The model under review builds one solid part; all positions refer to its coordinate system, in mm. A direction names the side the tool comes from. Give positions to 0.01 mm unless a question says otherwise; leave off trailing zeros. Write each loop counter-clockwise with the first axis right and the second up, starting at its lowest first coordinate (ties: lowest second). Pieces come first, ordered by that corner, then holes. Notation, with made-up numbers: (77.25, 44.25) - (113.25, 44.25) arc R19 cw to (113.25, 58.25) - close; hole circle Ø2 at (-8, 55). An arc over 180 degrees is marked (long way). Write item = value, one per line.
```python
from build123d import *

# Parameters (mm, degrees)
SALIENTE_EXTRUIR1_DEPTH                              = 10
PERFORADOR_PARA_ROSCAR_PARA_MACHO_DE_2_COUNT         = 2
PERFORADOR_PARA_ROSCAR_PARA_MACHO_DE_2_PITCH         = 50
PERFORADOR_PARA_ROSCAR_PARA_MACHO_DE_3_COUNT         = 2
PERFORADOR_PARA_ROSCAR_PARA_MACHO_DE_3_PITCH         = 114.274917137
PERFORADOR_PARA_ROSCAR_PARA_MACHO_DE_4_COUNT         = 2
PERFORADOR_PARA_ROSCAR_PARA_MACHO_DE_4_PITCH         = 25
PERFORADOR_PARA_ROSCAR_PARA_MACHO_DE_5_A_COUNT       = 2
PERFORADOR_PARA_ROSCAR_PARA_MACHO_DE_5_A_PITCH       = 50
PERFORADOR_PARA_ROSCAR_PARA_MACHO_DE_6_COUNT         = 2
PERFORADOR_PARA_ROSCAR_PARA_MACHO_DE_6_PITCH         = 24.875395913
REFRENTADO_PARA_TORNILLO_TAP_N_CON_CABEZ_D           = 5.3
REFRENTADO_PARA_TORNILLO_TAP_N_CON_CABEZ_CSINK_D     = 11.2
REFRENTADO_PARA_TORNILLO_TAP_N_CON_CABEZ_CSINK_ANGLE = 90
SIMETR_A3_COPY_1_D                                   = 5.3
SIMETR_A3_COPY_1_CSINK_D                             = 11.2
SIMETR_A3_COPY_1_CSINK_ANGLE                         = 90


with BuildPart() as part:
    # Croquis1 → Saliente-Extruir1 (new body)
    with BuildSketch(Plane.XY):
        with BuildLine():
            Line((-67.025, 50), (67.025, 50))
            ThreePointArc((67.025, 50), (91.773737342, 60.251262658), (102.025, 85))
            Line((102.025, 85), (102.025, 220))
            Line((102.025, 220), (182.025, 220))
            Line((182.025, 220), (182.025, 85.714285714))
            ThreePointArc((182.025, 85.714285714), (178.120745631, 66.344664275), (167.017710611, 50))
            ThreePointArc((167.017710611, 50), (146.007505467, 0), (167.017710611, -50))
            ThreePointArc((167.017710611, -50), (178.120745631, -66.344664275), (182.025, -85.714285714))
            Line((182.025, -85.714285714), (182.025, -220))
            Line((182.025, -220), (102.025, -220))
            Line((102.025, -220), (102.025, -85))
            ThreePointArc((102.025, -85), (91.773737342, -60.251262658), (67.025, -50))
            Line((67.025, -50), (-67.025, -50))
            ThreePointArc((-67.025, -50), (-91.773737342, -60.251262658), (-102.025, -85))
            Line((-102.025, -85), (-102.025, -220))
            Line((-102.025, -220), (-182.025, -220))
            Line((-182.025, -220), (-182.025, -85.714285714))
            ThreePointArc((-182.025, -85.714285714), (-178.120745631, -66.344664275), (-167.017710611, -50))
            ThreePointArc((-167.017710611, -50), (-146.007505467, 0), (-167.017710611, 50))
            ThreePointArc((-167.017710611, 50), (-178.120745631, 66.344664275), (-182.025, 85.714285714))
            Line((-182.025, 85.714285714), (-182.025, 220))
            Line((-182.025, 220), (-102.025, 220))
            Line((-102.025, 220), (-102.025, 85))
            ThreePointArc((-102.025, 85), (-91.773737342, 60.251262658), (-67.025, 50))
        make_face()
    extrude(amount=SALIENTE_EXTRUIR1_DEPTH)

    # Croquis3 → Perforador para roscar para macho de ros (revolve, cut)
    with BuildSketch(Plane(origin=(-167.025, 220, 5), x_dir=(0, 0, 1), z_dir=(1, 0, 0))):
        Polygon((0, 0), (0, 76.2618073), (2.1, 75), (2.1, 0), align=None)
    perforador_para_roscar_para_macho_de_ros = revolve(axis=Axis((-167.025, 226.35, 5), (0, -1, 0)), mode=Mode.SUBTRACT)

    # Perforador para roscar para macho de 2: Perforador para roscar para macho de ros ×2
    with Locations(*[(i * PERFORADOR_PARA_ROSCAR_PARA_MACHO_DE_2_PITCH, 0, 0) for i in range(1, PERFORADOR_PARA_ROSCAR_PARA_MACHO_DE_2_COUNT)]):
        add(perforador_para_roscar_para_macho_de_ros, mode=Mode.SUBTRACT)

    # Perforador para roscar para macho de 3: Perforador para roscar para macho de ros ×2
    with Locations(*[Vector(-0.9105437359751597, 0, -0.4134127536450694) * (i * PERFORADOR_PARA_ROSCAR_PARA_MACHO_DE_3_PITCH) for i in range(1, PERFORADOR_PARA_ROSCAR_PARA_MACHO_DE_3_COUNT)]):
        add(perforador_para_roscar_para_macho_de_ros, mode=Mode.SUBTRACT)

    # Perforador para roscar para macho de 4: Perforador para roscar para macho de ros ×2
    with Locations(*[(i * PERFORADOR_PARA_ROSCAR_PARA_MACHO_DE_4_PITCH, 0, 0) for i in range(1, PERFORADOR_PARA_ROSCAR_PARA_MACHO_DE_4_COUNT)]):
        add(perforador_para_roscar_para_macho_de_ros, mode=Mode.SUBTRACT)

    # Croquis5 → Perforador para roscar para macho de 5 (revolve, cut)
    with BuildSketch(Plane(origin=(117.025, 220, 5), x_dir=(0, 0, 1), z_dir=(1, 0, 0))):
        Polygon((0, 0), (0, 76.2618073), (2.1, 75), (2.1, 0), align=None)
    perforador_para_roscar_para_macho_de_5 = revolve(axis=Axis((117.025, 226.35, 5), (0, -1, 0)), mode=Mode.SUBTRACT)

    # Perforador para roscar para macho de 5 a: Perforador para roscar para macho de 5 ×2
    with Locations(*[(i * PERFORADOR_PARA_ROSCAR_PARA_MACHO_DE_5_A_PITCH, 0, 0) for i in range(1, PERFORADOR_PARA_ROSCAR_PARA_MACHO_DE_5_A_COUNT)]):
        add(perforador_para_roscar_para_macho_de_5, mode=Mode.SUBTRACT)

    # Perforador para roscar para macho de 6: Perforador para roscar para macho de 5 ×2
    with Locations(*[Vector(0.9999846303252095, 0, 0.005544286550521713) * (i * PERFORADOR_PARA_ROSCAR_PARA_MACHO_DE_6_PITCH) for i in range(1, PERFORADOR_PARA_ROSCAR_PARA_MACHO_DE_6_COUNT)]):
        add(perforador_para_roscar_para_macho_de_5, mode=Mode.SUBTRACT)

    # Simetría1: Perforador para roscar para macho de ros, Perforador para roscar para macho de 5 across plane
    add(perforador_para_roscar_para_macho_de_ros.mirror(Plane.ZX), mode=Mode.SUBTRACT)
    add(perforador_para_roscar_para_macho_de_5.mirror(Plane.ZX), mode=Mode.SUBTRACT)

    # Simetría1 copy 1 sketch → Simetría1 copy 1 (revolve, cut)
    with BuildSketch(Plane(origin=(-117.025, -220, 5), x_dir=(0, 0, 1), z_dir=(1, 0, 0))):
        Polygon((0, 0), (0, -76.2618073), (2.1, -75), (2.1, 0), align=None)
    revolve(axis=Axis((-117.025, -226.35, 5), (0, -1, 0)), mode=Mode.SUBTRACT)

    # Simetría1 copy 2 sketch → Simetría1 copy 2 (revolve, cut)
    with BuildSketch(Plane(origin=(-271.077309978, -220, -42.242708166), x_dir=(0, 0, 1), z_dir=(1, 0, 0))):
        Polygon((0, 0), (0, -76.2618073), (2.1, -75), (2.1, 0), align=None)
    revolve(axis=Axis((-271.077309978, -226.35, -42.242708166), (0, -1, 0)), mode=Mode.SUBTRACT)

    # Simetría1 copy 3 sketch → Simetría1 copy 3 (revolve, cut)
    with BuildSketch(Plane(origin=(-142.025, -220, 5), x_dir=(0, 0, 1), z_dir=(1, 0, 0))):
        Polygon((0, 0), (0, -76.2618073), (2.1, -75), (2.1, 0), align=None)
    revolve(axis=Axis((-142.025, -226.35, 5), (0, -1, 0)), mode=Mode.SUBTRACT)

    # Simetría1 copy 4 sketch → Simetría1 copy 4 (revolve, cut)
    with BuildSketch(Plane(origin=(167.025, -220, 5), x_dir=(0, 0, 1), z_dir=(1, 0, 0))):
        Polygon((0, 0), (0, -76.2618073), (2.1, -75), (2.1, 0), align=None)
    revolve(axis=Axis((167.025, -226.35, 5), (0, -1, 0)), mode=Mode.SUBTRACT)

    # Simetría1 copy 5 sketch → Simetría1 copy 5 (revolve, cut)
    with BuildSketch(Plane(origin=(141.900013587, -220, 5.137916323), x_dir=(0, 0, 1), z_dir=(1, 0, 0))):
        Polygon((0, 0), (0, -76.2618073), (2.1, -75), (2.1, 0), align=None)
    revolve(axis=Axis((141.900013587, -226.35, 5.137916323), (0, -1, 0)), mode=Mode.SUBTRACT)

    # Refrentado para tornillo tapón con cabeza plana de clavija de M51 (through all)
    with Locations(Plane(origin=(148.520190528, -141, 0), x_dir=(-1, 0, 0), z_dir=(0, 0, -1))):
        with Locations((0, 0), (12.990381056, 7.5), (12.990381056, -7.5), (0, 15)):
            refrentado_para_tornillo_tap_n_con_cabez = CounterSinkHole(REFRENTADO_PARA_TORNILLO_TAP_N_CON_CABEZ_D / 2, REFRENTADO_PARA_TORNILLO_TAP_N_CON_CABEZ_CSINK_D / 2, counter_sink_angle=REFRENTADO_PARA_TORNILLO_TAP_N_CON_CABEZ_CSINK_ANGLE)

    # Simetría2: Refrentado para tornillo tapón con cabeza plana de clavija de M51 across plane
    add(refrentado_para_tornillo_tap_n_con_cabez.mirror(Plane.ZX), mode=Mode.SUBTRACT)

    # Simetría3: Refrentado para tornillo tapón con cabeza plana de clavija de M51 across plane
    add(refrentado_para_tornillo_tap_n_con_cabez.mirror(Plane(origin=(0, 0, 0), x_dir=(0, 0, 1), z_dir=(1, 0, 0))), mode=Mode.SUBTRACT)

    # Simetría3 copy 1 (through all)
    with Locations(Plane(origin=(-148.520190528, 141, 0), x_dir=(1, 0, 0), z_dir=(0, 0, -1))):
        with Locations((0, 0), (12.990381056, 7.5), (12.990381056, -7.5), (0, 15)):
            CounterSinkHole(SIMETR_A3_COPY_1_D / 2, SIMETR_A3_COPY_1_CSINK_D / 2, counter_sink_angle=SIMETR_A3_COPY_1_CSINK_ANGLE)


solid = part.part
```
1. For line 1 (X direction, y = 141, z = 5.5) (3 decimals); line 2 (X direction, y = 141, z = 2.5) (3 decimals); line 3 (Y direction, x = -134, z = 6), list the stretches that pass through material, from the lowest coordinate up. Write a range as from..to.
Findings below:
line_1 = -182.025..-151.17, -145.87..-102.025, 102.025..145.87, 151.17..182.025
line_2 = -182.025..-151.62, -145.42..-102.025, 102.025..145.42, 151.62..182.025
line_3 = -220..-150.66, -146.34..-135.66, -131.34..131.34, 135.66..146.34, 150.66..220
2. Take a section at B-B on x = -28. Give the boundary of the cut face in (y, z), and give its area (3 significant figures).
Findings below:
outline = (-50, 0) - (50, 0) - (50, 10) - (-50, 10) - close
area = 1,000 mm²
3. Draft analysis for pull direction X (two halves, no side actions). For faces 1 (the flat face through (3, 3, 0)), 2 (the conical face through (-135.166, 130.731, 2.807)), 3 (the cylindrical face through (178.228, 66.602, 4.93)), state which applies: +X half, -X half, draft (parallel to the pull), parting line (faces both ways), or undercut.
Findings below:
face_1 = draft
face_2 = undercut
face_3 = +X half
4. Machinability: for faces 4 (the flat face through (102.025, -153, 5)), 5 (the cylindrical face through (-178.228, -66.602, 4.93)), 6 (the conical face through (151.18, -140.16, 2.81)), 7 (the cylindrical face through (-92.04, 60.52, 4.93)), which of the approach directions +Z, -Z, +X, -X, +Y, -Y give a long, thin tool a straight path to every point of the face, cutting with its end or side? Answer none if there is none.
Findings below:
face_4 = +Z, -Z, -Y
face_5 = +Z, -Z, -X
face_6 = -Z
face_7 = +Z, -Z, +Y
5. Insertion check: P1, Ø3.5, axis at x = 117.025, z = 5, coming from the +Y side; P2, Ø5, axis at x = 28, z = 4, coming from the -Y side; P3, Ø6, axis at x = 135.53, y = 133.5, coming from the -Z side. Each pin has a flat end and moves straight along its axis. Give the tip position at first contact, or say it passes through.
Findings below:
P1 = 144.79
P2 = -50
P3 = 2.6
6. Take a section at A-A on y = -63.5. Give the boundary of the cut face in (x, z).
Findings below:
outline = (-176.82, 0) - (-94.64, 0) - (-94.64, 10) - (-176.82, 10) - close; (94.64, 0) - (176.82, 0) - (176.82, 10) - (94.64, 10) - close
